from build123d import *

# Parameters (mm, degrees)
F0_W     = 6
F0_H     = 353
F1_DEPTH = 1.5
F2_W     = 6
F2_H     = 353
F2_W_2   = 3
F2_H_2   = 350
F3_DEPTH = 10
F5_DEPTH = 100
F6_W     = 228.872508
F6_H     = 47.288619
F7_DEPTH = 25


with BuildPart() as f1:
    # F0 (on Top) → F1 (new body)
    with BuildSketch(Plane.XY):
        Rectangle(F0_W, F0_H)
    extrude(amount=F1_DEPTH)

    # F2 (on face) → F3 (join)
    with BuildSketch(Plane.XY.offset(1.5)):
        Rectangle(F2_W, F2_H)
        Rectangle(F2_W_2, F2_H_2, mode=Mode.SUBTRACT)
    extrude(amount=F3_DEPTH)

    # F4 (on face) → F5 (join)
    with BuildSketch(Plane.XY.offset(11.5)):
        Polygon((1.5, -175), (-1.5, -175), (-1.5, -165), (-3, -165), (-3, -176.5), (3, -176.5), (3, -165), (1.5, -165), align=None)
    extrude(amount=F5_DEPTH)

    # F6 (on face) → F7 (cut)
    with BuildSketch(Plane.YZ.offset(3)):
        with Locations((114.436254, 23.644309)):
            Rectangle(F6_W, F6_H)
    extrude(amount=-F7_DEPTH, mode=Mode.SUBTRACT)

    # F8: F1 across plane


with BuildPart() as f1_1:
    add(f1.part)
    add(f1.part.mirror(Plane.XZ))


solid = f1_1.part
Here's how the part is built. I have some questions about the finished solid (model axes, mm). A direction names the side the tool comes from. Coordinates: 2 decimals unless noted, no trailing zeros. Order: outer loops, then holes, each group sorted by start corner. A loop starts at its lowest first (then second) coordinate and runs counter-clockwise, first axis right, second up. Notation, with made-up numbers: (70.25, 9.25) - (87.25, 9.25) arc R13 cw to (87.25, 24.25) - close; hole circle Ø3 at (43, 64). An arc over 180 degrees is marked (long way). Use CSV: the item, a comma, the result in double quotes. Start each with the question number.
1. Please list where these lines run through material, in increasing order: line 1 (X direction, y = 102.5, z = 11); line 2 (Y direction, x = 0.85, z = 88); line 3 (Y direction, x = -2.7, z = 26). Write a range as from..to.
2. Suppose I cut it at A-A on z = 70. List the corners of the cut face in (x, y) for me.
3. For faces 1 (the face through (-2, -171, 111.5)), 2 (the face through (-1.5, 1, 11)), which set-ups out of +Z, -Z, +X, -X, +Y, -Y let a thin tool reach every point of the face, with its end or its side?
4. Suppose I cut it at C-C on x = 0.3. List the corners of the cut face in (y, z) for me.
5. Suppose I cut it at B-B on y = 134. List the corners of the cut face in (x, z) for me, then the cut area to 3 significant figures.
6. I'm going to push flat-ended pins straight in: pin 1 (1.6 mm diameter, centred on x = -2, y = -74, fed in from +Z); pin 2 (2 mm diameter, centred on x = 0, y = 42, fed in from +Z). Where does each tip first touch, or does it pass through?
Output:
1,line 1,"x = -3..-1.5, 1.5..3"
1,line 2,"y = -176.5..-175, 175..176.5"
1,line 3,"y = -176.5..-165, 165..176.5"
2,outline,"(-3, -176.5) - (3, -176.5) - (3, -165) - (1.5, -165) - (1.5, -175) - (-1.5, -175) - (-1.5, -165) - (-3, -165) - close; (-3, 165) - (-1.5, 165) - (-1.5, 175) - (1.5, 175) - (1.5, 165) - (3, 165) - (3, 176.5) - (-3, 176.5) - close"
3,face 1,"+Z, +X, -X, +Y, -Y"
3,face 2,"+Z"
4,outline,"(-176.5, 0) - (176.5, 0) - (176.5, 111.5) - (175, 111.5) - (175, 1.5) - (-175, 1.5) - (-175, 111.5) - (-176.5, 111.5) - close"
5,outline,"(-3, 0) - (3, 0) - (3, 11.5) - (1.5, 11.5) - (1.5, 1.5) - (-1.5, 1.5) - (-1.5, 11.5) - (-3, 11.5) - close"
5,area,"39.0 mm2"
6,pin 1,"stops at z = 11.5"
6,pin 2,"stops at z = 1.5"
